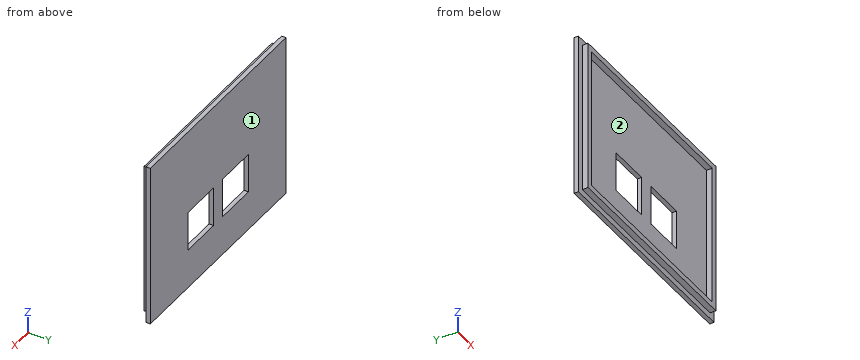
from build123d import *

# Parameters (mm, degrees)
IZIM1_W                     = 74
IZIM1_H                     = 58
Y_KSEKLIK_EKSTR_ZYON1_DEPTH = 1.5
IZIM2_W                     = 69.8
IZIM2_H                     = 53.8
IZIM2_W_2                   = 65.8
IZIM2_H_2                   = 49.8
EKSTR_ZYON_NCE1_DEPTH       = 2
IZIM4_W                     = 14
IZIM4_H                     = 14
KES_EKSTR_ZYON4_DEPTH       = 2


with BuildPart() as part:
    # Çizim1 → Yükseklik-Ekstrüzyon1 (new body)
    with BuildSketch(Plane(origin=(0, 0, 0), x_dir=(1, 0, 0), z_dir=(0, 1, 0))):
        Rectangle(IZIM1_W, IZIM1_H)
    extrude(amount=Y_KSEKLIK_EKSTR_ZYON1_DEPTH)

    # Çizim2 → Ekstrüzyon-İnce1 (add)
    with BuildSketch(Plane.XZ):
        Rectangle(IZIM2_W, IZIM2_H)
        Rectangle(IZIM2_W_2, IZIM2_H_2, mode=Mode.SUBTRACT)
    extrude(amount=EKSTR_ZYON_NCE1_DEPTH)

    # Çizim4 → Kes-Ekstrüzyon4 (cut)
    with BuildSketch(Plane(origin=(0, 1.5, 0), x_dir=(1, 0, 0), z_dir=(0, 1, 0))):
        with Locations((-9.525, 8)):
            Rectangle(IZIM4_W, IZIM4_H)
        with Locations((9.525, 8)):
            Rectangle(IZIM4_W, IZIM4_H)
    extrude(amount=-KES_EKSTR_ZYON4_DEPTH, mode=Mode.SUBTRACT)


solid = part.part
Can you work these out from the model? Positions are in its coordinate system, mm. Face numbers are marked on the shaded views. Coordinates: 2 decimals unless noted, no trailing zeros. Order: outer loops, then holes, each group sorted by start corner. A loop starts at its lowest first (then second) coordinate and runs counter-clockwise, first axis right, second up. Notation, with made-up numbers: M 46,-32.5 L 52,-32.5 A16 ccw 52,-7.5 Z; hole C 3.25,38 d2. An arc over 180 degrees is marked long. Answer as CSV lines item,"result".
(1) Please list where these lines run through material, in increasing order: L1, parallel to X at y = 0.35, z = -4 (3 decimals); L2, parallel to Z at x = -26, y = -0.65; L3, parallel to X at y = -0.1, z = 21.5.
Geometry check:
L1,"-37 to -16.525, -2.525 to 2.525, 16.525 to 37"
L2,"-26.9 to -24.9, 24.9 to 26.9"
L3,"-34.9 to -32.9, 32.9 to 34.9"
(2) Suppose I cut it at C-C on y = -1.35. Please give me the cut outline in (x, z), plus the area to 3 significant figures.
Geometry check:
outline,"M -34.9,-26.9 L 34.9,-26.9 L 34.9,26.9 L -34.9,26.9 Z; hole M -32.9,-24.9 L 32.9,-24.9 L 32.9,24.9 L -32.9,24.9 Z"
area,"478 mm^2"
(3) I'm going to push flat-ended pins straight in: pin 1 (2 mm diameter, centred on x = -8, y = -1.5, fed in from +Z); pin 2 (1 mm diameter, centred on y = -1, z = -0.5, fed in from -X); pin 3 (1.6 mm diameter, centred on x = 0, y = -1, fed in from -Z). Where does each tip first touch, or does it pass through?
Geometry check:
pin 1,"z = 26.9"
pin 2,"x = -34.9"
pin 3,"z = -26.9"
(4) Suppose I cut it at D-D on x = 27. Please give me the cut outline in (y, z), plus the area to 3 significant figures.
Geometry check:
outline,"M -2,-26.9 L 0,-26.9 L 0,-29 L 1.5,-29 L 1.5,29 L 0,29 L 0,26.9 L -2,26.9 L -2,24.9 L 0,24.9 L 0,-24.9 L -2,-24.9 Z"
area,"95.0 mm^2"
(5) Suppose I cut it at A-A on z = -13.5. Please give me the cut outline in (x, y) (3 decimals).
Geometry check:
outline,"M -37,0 L -34.9,0 L -34.9,-2 L -32.9,-2 L -32.9,0 L -16.525,0 L -16.525,1.5 L -37,1.5 Z; M -2.525,0 L 2.525,0 L 2.525,1.5 L -2.525,1.5 Z; M 16.525,0 L 32.9,0 L 32.9,-2 L 34.9,-2 L 34.9,0 L 37,0 L 37,1.5 L 16.525,1.5 Z"
(6) If we mould it in two halves opening along X, with no side actions, what happens to the marked faces 1 and 2? For each: released by +X, released by -X, zero draft, split by the parting line, or undercut.
Geometry check:
face 1,"zero draft"
face 2,"undercut"
(7) Suppose I cut it at B-B on x = 5. Please give me the cut outline in (y, z).
Geometry check:
outline,"M -2,-26.9 L 0,-26.9 L 0,-29 L 1.5,-29 L 1.5,-15 L 0,-15 L 0,-24.9 L -2,-24.9 Z; M -2,24.9 L 0,24.9 L 0,-1 L 1.5,-1 L 1.5,29 L 0,29 L 0,26.9 L -2,26.9 Z"
